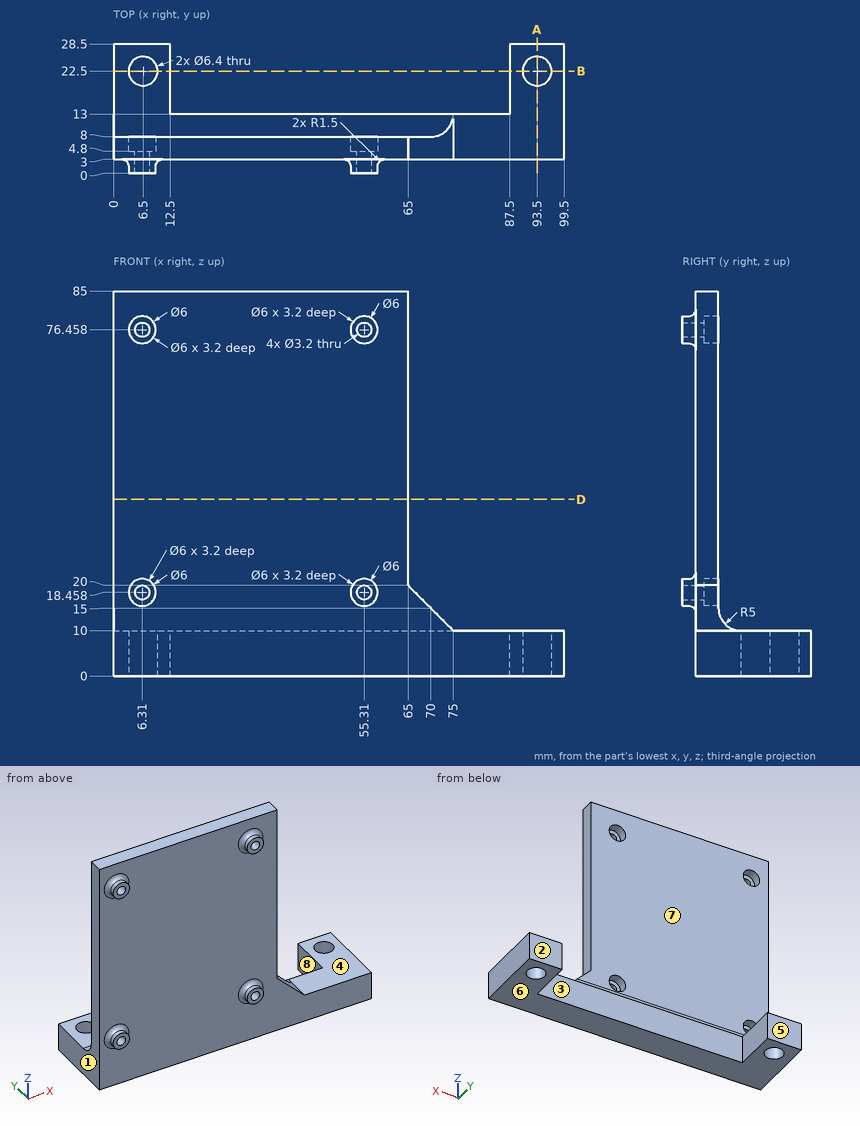
Geometry: see drawing. Coordinates: mm, zero at the bounding-box minimum. A direction names the side the tool comes from. Give positions to 0.01 mm unless a question says otherwise; leave off trailing zeros. Order: outer loops, then holes, each group sorted by start corner. A loop starts at its lowest first (then second) coordinate and runs counter-clockwise, first axis right, second up. Notation, with made-up numbers: (61, 27) - (86, 27) arc R20 cw to (86, 54) - close; hole circle Ø10 at (-17.75, 13.25). An arc over 180 degrees is marked (long way). Use a Markdown table: item, result.
(1) Draft query along X for the marked faces 1, 2 and 3. Return one class per face: released by +X, released by -X, zero draft, split by the parting line, or undercut.
Computed values:
| item | result |
|---|---|
| face 1 | released by -X |
| face 2 | zero draft |
| face 3 | undercut |
(2) Section query D-D (z = 39). Output: boundary loops of the cut face in (x, y).
Computed values:
| item | result |
|---|---|
| outline | (0, 3) - (65, 3) - (65, 8) - (0, 8) - close |
(3) Line query: line 1 (Z direction, x = 4, y = 5) (1 decimal); line 2 (X direction, y = 26.25, z = 6); line 3 (Y direction, x = 93.5, z = 5). Output: solid intervals per line, ascending. Write a range as from..to.
Computed values:
| item | result |
|---|---|
| line 1 | z = 0..16.5, 20.4..74.5, 78.4..85 |
| line 2 | x = 0..12.5, 87.5..99.5 |
| line 3 | y = 3..19.3, 25.7..28.5 |
(4) Section query B-B (y = 22.5). Output: boundary loops of the cut face in (x, z), then the cut area to 3 significant figures.
Computed values:
| item | result |
|---|---|
| outline | (0, 0) - (3.3, 0) - (3.3, 10) - (0, 10) - close; (9.7, 0) - (12.5, 0) - (12.5, 10) - (9.7, 10) - close; (87.5, 0) - (90.3, 0) - (90.3, 10) - (87.5, 10) - close; (96.7, 0) - (99.5, 0) - (99.5, 10) - (96.7, 10) - close |
| area | 117 mm2 |
(5) Section query A-A (x = 93.5). Output: boundary loops of the cut face in (y, z).
Computed values:
| item | result |
|---|---|
| outline | (3, 0) - (19.3, 0) - (19.3, 10) - (3, 10) - close; (25.7, 0) - (28.5, 0) - (28.5, 10) - (25.7, 10) - close |
(6) Access query for the marked faces 4, 5, 6, 7 and 8. Directions: +Z, -Z, +X, -X, +Y, -Y. A direction counts if a zero-diameter tool reaches every point of the face in a straight line with its end or side. Return the directions, or none.
Computed values:
| item | result |
|---|---|
| face 4 | +Z, +X, +Y, -Y |
| face 5 | +Z, -Z, +X, -X, +Y |
| face 6 | -Z, +X, -X, +Y, -Y |
| face 7 | +Z, +X, -X, +Y |
| face 8 | +Z, -Z, +Y |
(7) Pin query (flat end, axial travel): pin 1 (8 mm diameter, centred on x = 78, y = 8, fed in from +Z); pin 2 (5 mm diameter, centred on x = 6.31, z = 18.46, fed in from +Y); pin 3 (1 mm diameter, centred on x = 18.5, z = 47.5, fed in from -Y); pin 4 (5 mm diameter, centred on x = 93.5, y = 22.5, fed in from -Z). Return the tip coordinate at first contact, or that it passes through.
Computed values:
| item | result |
|---|---|
| pin 1 | stops at z = 11 |
| pin 2 | stops at y = 4.8 |
| pin 3 | stops at y = 3 |
| pin 4 | passes through |
